Design review of the part built by this model. Coordinates are the model's own, in mm. A direction names the side the tool comes from. Coordinates: 2 decimals unless noted, no trailing zeros. Write each loop counter-clockwise with the first axis right and the second up, starting at its lowest first coordinate (ties: lowest second). Pieces come first, ordered by that corner, then holes. Notation, with made-up numbers: (16, -4.75) -> (28, -4.75) arc R8 ccw to (28, 9.25) -> close; hole circle Ø11 at (71.5, -39.5). An arc over 180 degrees is marked (long way). Write item = value, one per line. Start each with the question number.
```python
from build123d import *

# Parameters (mm, degrees)
F2_R     = 5
F3_R     = 11
F4_DEPTH = 30


with BuildPart() as f1:
    # F0 (on Top) → F1 (revolve)
    with BuildSketch(Plane.XY):
        Polygon((-222.5, 0), (-150, 0), (-150, 125), (-161.95, 118.100664), (-161.95, 78.100664), (-171.31308, 25), (-222.5, 25), align=None)
    revolve(axis=Axis((0, 128.547966, 0), (0, 1, 0)))

    # F2
    f2_edges = [f1.edges().sort_by_distance(p)[0] for p in [
        (171.31308, 25, 0),
        (161.95, 78.100664, 0),
    ]]
    fillet(f2_edges, radius=F2_R)

    # F3 (on face) → F4 (cut)
    with BuildSketch(Plane(origin=(0, 25, 0), x_dir=(-1, 0, 0), z_dir=(0, 1, 0))):
        with Locations((108.713881, -167.872845)):
            Circle(F3_R)
        with Locations((178.085405, -91.025207)):
            Circle(F3_R)
        with Locations((199.739089, 10.212561)):
            Circle(F3_R)
        with Locations((167.872845, 108.713881)):
            Circle(F3_R)
        with Locations((91.025207, 178.085405)):
            Circle(F3_R)
        with Locations((-10.212561, 199.739089)):
            Circle(F3_R)
        with Locations((-108.713881, 167.872845)):
            Circle(F3_R)
        with Locations((-178.085405, 91.025207)):
            Circle(F3_R)
        with Locations((-199.739089, -10.212561)):
            Circle(F3_R)
        with Locations((-167.872845, -108.713881)):
            Circle(F3_R)
        with Locations((-91.025207, -178.085405)):
            Circle(F3_R)
        with Locations((10.212561, -199.739089)):
            Circle(F3_R)
    extrude(amount=-F4_DEPTH, mode=Mode.SUBTRACT)


solid = f1.part
```
(1) Take a section at B-B, the plane y = 40. State the section outline as (x, z) points.
(2) Take a section at A-A, the plane y = 94. State the section outline as (x, z) points, then the cut area to 3 significant figures.
(3) For pin 1 Ø8 at (x, y) = (136, 76) entering from +Z; pin 2 Ø4 at (x, y) = (140.5, 63.5) entering from -Z; pin 3 Ø10 at (y, z) = (57.5, -141) entering from +X, all flat-tipped, find the tip position at first contact; note any pin that passes through.
(4) For line 1 (X direction, y = 101.5, z = -137); line 2 (X direction, y = 82, z = 12.5); line 3 (Z direction, x = -55, y = 67), list the stretches that pass through material, from the lowest coordinate up.
(5) Mouldability with a two-part tool opening along X and no side actions: class faces 3 (the face through (28.965, 12.325, 220.607)), 4 (the face through (-119.206, 12.675, -164.569)), 5 (the face through (-67, 25, -164)) as pulls with the +X half, pulls with the -X half, needs draft (parallel to the pull), parting line crosses it, or undercut.
(6) For faces 1 (the face through (178.862, 12.675, -108.23)), 2 (the face through (35.1, 98, -158.1)), list the 3-axis set-ups (+Z, -Z, +X, -X, +Y, -Y) from which the entire face can be reached by the end or side of a thin tool; tool diameter is ignored.
Report:
q1.outline = circle Ø337.34 at (0, 0); hole circle Ø300 at (0, 0)
q2.outline = circle Ø323.9 at (0, 0); hole circle Ø300 at (0, 0)
q2.area = 11,700 mm2
q3.pin_1 = 94.6
q3.pin_2 = -88.87
q3.pin_3 = 94.62
q4.line_1 = -86.36 to -61.08, 61.08 to 86.36
q4.line_2 = -161.47 to -149.48, 149.48 to 161.47
q4.line_3 = -154.4 to -139.55, 139.55 to 154.4
q5.face_3 = parting line crosses it
q5.face_4 = undercut
q5.face_5 = needs draft
q6.face_1 = +Y, -Y
q6.face_2 = +Y
